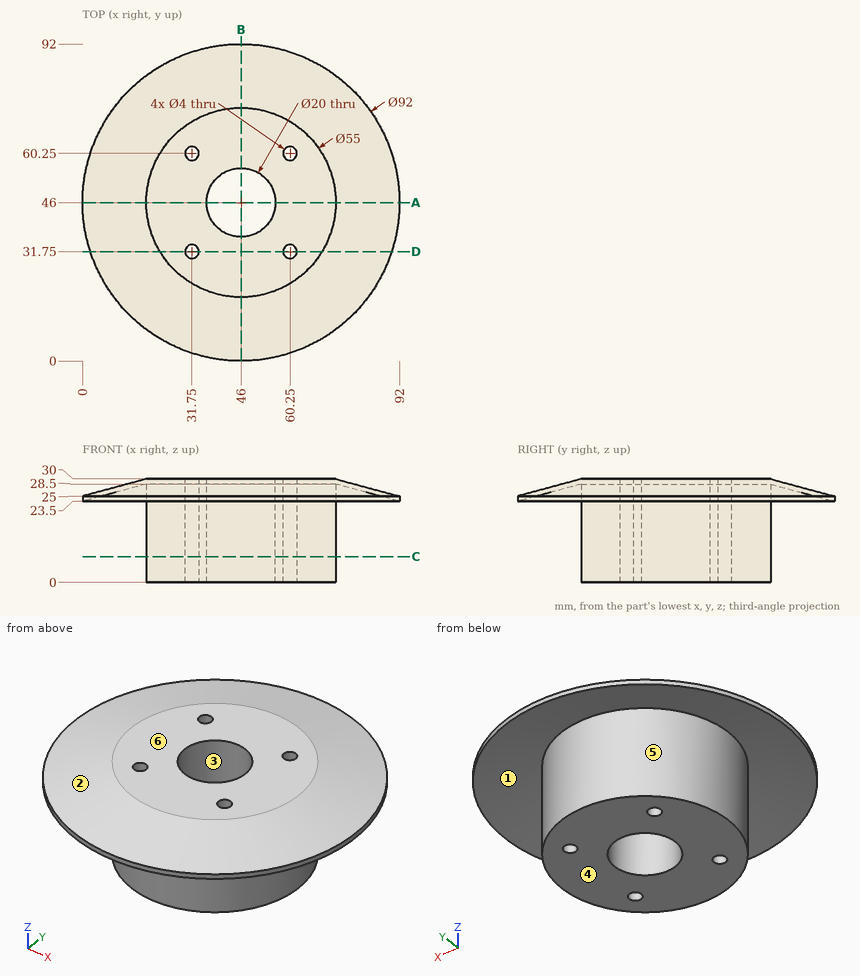
Geometry check sheet. Reference: drawing and pictorial views, mm from the part's lowest x, y, z. A direction names the side the tool comes from. Round coordinates to 2 decimals unless told otherwise and drop trailing zeros. Write each loop counter-clockwise with the first axis right and the second up, starting at its lowest first coordinate (ties: lowest second). Pieces come first, ordered by that corner, then holes.
1. Section check D-D on y = 31.75. State how many separate pieces and enclosed holes the cut face has, plus the area to 3 significant figures.
2. Section check C-C on z = 7.5. Enter the section's corners in (x, y).
3. Access from +Z, -Z, +X, -X, +Y, -Y to the whole of each face (thin tool, end or side, straight path). Record for the marked faces 5 and 6.
4. Draft check along Y on the marked faces 1, 2, 3 and 4. Enter one of: +Y half, -Y half, draft (parallel to the pull), parting line (faces both ways), or undercut.
5. Gauge pin test, flat ends, axial feed: P1, Ø12, axis at x = 30, z = 25.5, coming from the +Y side; P2, Ø8, axis at x = 51, y = 16.5, coming from the +Z side; P3, Ø12, axis at x = 82.5, y = 71, coming from the -Z side; P4, Ø1, axis at x = 45, z = 19, coming from the +Y side. Record the tip position at first contact, or that the pin passes through.
6. Section check A-A on y = 46. Enter the section's corners in (x, z), plus the area to 3 significant figures.
7. Scan lines: L1, parallel to Y at x = 60.25, z = 18.75; L2, parallel to X at y = 46, z = 13.75. Record each from-to range of solid material in increasing order.
Answer:
1. separate pieces: 3
1. enclosed holes: 0
1. area: 1,230 mm2
2. outline: circle Ø55 at (46, 46); hole circle Ø4 at (31.75, 31.75); hole circle Ø4 at (31.75, 60.25); hole circle Ø20 at (46, 46); hole circle Ø4 at (60.25, 31.75); hole circle Ø4 at (60.25, 60.25)
3. face 5: -Z
3. face 6: +Z, +X, -X, +Y, -Y
4. face 1: undercut
4. face 2: parting line
4. face 3: undercut
4. face 4: draft
5. P1: stops at y = 90.9
5. P2: stops at z = 30
5. P3: stops at z = 23.5
5. P4: stops at y = 73.5
6. outline: (0, 23.5) - (18.5, 28.5) - (18.5, 0) - (36, 0) - (36, 30) - (18.5, 30) - (0, 25) - close; (56, 0) - (73.5, 0) - (73.5, 28.5) - (92, 23.5) - (92, 25) - (73.5, 30) - (56, 30) - close
6. area: 1,110 mm2
7. L1: y = 22.48 to 29.75, 33.75 to 58.25, 62.25 to 69.52
7. L2: x = 18.5 to 36, 56 to 73.5
